CAD build for the part. Positions are in the model's coordinates, mm. Face numbers are marked on the shaded views. A direction names the side the tool comes from. Give positions to 0.01 mm unless a question says otherwise; leave off trailing zeros. Write each loop counter-clockwise with the first axis right and the second up, starting at its lowest first coordinate (ties: lowest second). Pieces come first, ordered by that corner, then holes. Notation, with made-up numbers: (-10, 46.25) - (35, 46.25) arc R12 cw to (35, 53.25) - close; hole circle Ø7 at (87.5, -28). An arc over 180 degrees is marked (long way). Answer as a JSON object with one key per item and string values.
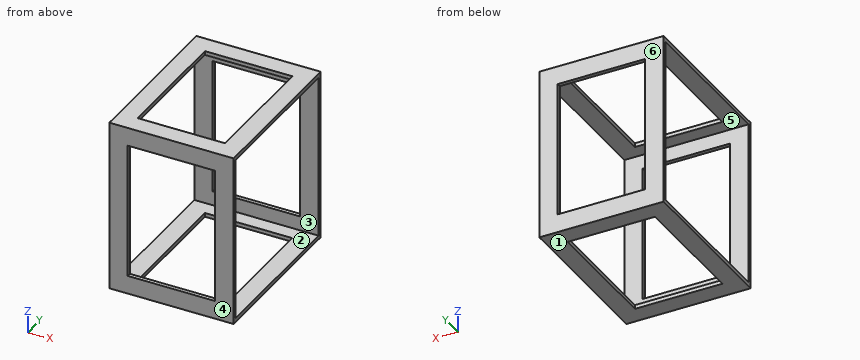
from build123d import *

# Parameters (mm, degrees)
SKETCH_W        = 782.5
SKETCH_H        = 833.8
SKETCH_W_2      = 744.4
SKETCH_H_2      = 795.7
PAD_DEPTH       = 600
SKETCH001_W     = 656
SKETCH001_H     = 422.2
POCKET_DEPTH    = 782.501
SKETCH002_W     = 604.7
SKETCH002_H     = 422.2
POCKET001_DEPTH = 833.801


with BuildPart() as part:
    # Sketch → Pad (new body)
    with BuildSketch(Plane.YZ):
        with Locations((-391.25, 416.9)):
            Rectangle(SKETCH_W, SKETCH_H)
        with Locations((-391.25, 416.9)):
            Rectangle(SKETCH_W_2, SKETCH_H_2, mode=Mode.SUBTRACT)
    extrude(amount=PAD_DEPTH)

    # Sketch001 (on Face4 of Pad) → Pocket (cut, through all)
    with BuildSketch(Plane(origin=(0, -782.5, 0), x_dir=(0, 0, -1), z_dir=(0, -1, 0))):
        with Locations((-416.9, 300)):
            Rectangle(SKETCH001_W, SKETCH001_H)
    extrude(amount=-POCKET_DEPTH, mode=Mode.SUBTRACT)

    # Sketch002 (on Face1 of Pocket) → Pocket001 (cut, through all)
    with BuildSketch(Plane(origin=(0, 0, 833.8), x_dir=(0, -1, 0), z_dir=(0, 0, 1))):
        with Locations((391.25, 300)):
            Rectangle(SKETCH002_W, SKETCH002_H)
    extrude(amount=-POCKET001_DEPTH, mode=Mode.SUBTRACT)


solid = part.part
(1) Saw through at A-A, the plane x = 373. Give the cut face in (y, z).
Answer key:
{"outline": "(-782.5, 0) - (-693.6, 0) - (-693.6, 19.05) - (-763.45, 19.05) - (-763.45, 88.9) - (-782.5, 88.9) - close; (-782.5, 744.9) - (-763.45, 744.9) - (-763.45, 814.75) - (-693.6, 814.75) - (-693.6, 833.8) - (-782.5, 833.8) - close; (-88.9, 0) - (0, 0) - (0, 88.9) - (-19.05, 88.9) - (-19.05, 19.05) - (-88.9, 19.05) - close; (-88.9, 814.75) - (-19.05, 814.75) - (-19.05, 744.9) - (0, 744.9) - (0, 833.8) - (-88.9, 833.8) - close"}
(2) Saw through at B-B, the plane y = -315. Give the cut face in (x, z), and give its area (3 significant figures).
Answer key:
{"outline": "(0, 0) - (88.9, 0) - (88.9, 19.05) - (0, 19.05) - close; (0, 814.75) - (88.9, 814.75) - (88.9, 833.8) - (0, 833.8) - close; (511.1, 0) - (600, 0) - (600, 19.05) - (511.1, 19.05) - close; (511.1, 814.75) - (600, 814.75) - (600, 833.8) - (511.1, 833.8) - close", "area": "6,770 mm²"}
(3) Pull direction Y, two halves, no side cores. Call the marked faces 3, 4, 5 and 6: pulls with the +Y half, pulls with the -Y half, needs draft (parallel to the pull), parting line crosses it, or undercut.
Answer key:
{"face 3": "undercut", "face 4": "pulls with the -Y half", "face 5": "undercut", "face 6": "pulls with the +Y half"}
(4) 3-axis set-ups, long thin cutter, end or side, ignore diameter. For the marked faces 1 and 2: which of +Z, -Z, +X, -X, +Y, -Y reach the whole face in a straight line?
Answer key:
{"face 1": "-Z, +X, -X, +Y, -Y", "face 2": "+X, -X"}
(5) Saw through at D-D, the plane x = 40.5. Give the cut face in (y, z).
Answer key:
{"outline": "(-782.5, 0) - (0, 0) - (0, 833.8) - (-782.5, 833.8) - close; hole (-763.45, 19.05) - (-19.05, 19.05) - (-19.05, 814.75) - (-763.45, 814.75) - close"}
(6) Probe L1, parallel to Y at x = 379, z = 35.5; L2, parallel to Z at x = 297.5, y = -84. List the from-to ranges inside material, lowest first. Write a range as [from, to].
Answer key:
{"L1": "y = [-782.5, -763.45], [-19.05, 0]", "L2": "z = [0, 19.05], [814.75, 833.8]"}
(7) Saw through at C-C, the plane z = 722.5. Give the cut face in (x, y), and give its area (3 significant figures).
Answer key:
{"outline": "(0, -782.5) - (88.9, -782.5) - (88.9, -763.45) - (0, -763.45) - close; (0, -19.05) - (88.9, -19.05) - (88.9, 0) - (0, 0) - close; (511.1, -782.5) - (600, -782.5) - (600, -763.45) - (511.1, -763.45) - close; (511.1, -19.05) - (600, -19.05) - (600, 0) - (511.1, 0) - close", "area": "6,770 mm²"}
